Input: part model. Units: mm. Frame: model coordinates. Round coordinates to 2 decimals unless told otherwise and drop trailing zeros. Write each loop counter-clockwise with the first axis right and the second up, starting at its lowest first coordinate (ties: lowest second). Pieces come first, ordered by that corner, then holes. Notation, with made-up numbers: (17, 17) - (68, 17) arc R13 cw to (68, 26) - close; hole circle Ø9 at (61, 4). An arc over 180 degrees is marked (long way). Use one line per item in the form item = value.
```python
from build123d import *

# Parameters (mm, degrees)
SKETCH1_W           = 128
SKETCH1_H           = 90
SKETCH1_R           = 2.4
SKETCH1_R_2         = 1.5
BOSS_EXTRUDE3_DEPTH = 10


with BuildPart() as part:
    # Sketch1 → Boss-Extrude3 (new body)
    with BuildSketch(Plane.XY):
        with Locations((-55.79, 35.875)):
            Rectangle(SKETCH1_W, SKETCH1_H)
        with Locations((0, 71.73)):
            Circle(SKETCH1_R, mode=Mode.SUBTRACT)
        with Locations((-111.58, 0)):
            Circle(SKETCH1_R, mode=Mode.SUBTRACT)
        Circle(SKETCH1_R, mode=Mode.SUBTRACT)
        with Locations((-111.58, 71.73)):
            Circle(SKETCH1_R, mode=Mode.SUBTRACT)
        with Locations((-97.694375804, 60.375)):
            Circle(SKETCH1_R_2, mode=Mode.SUBTRACT)
        with Locations((-39.694375804, 60.375)):
            Circle(SKETCH1_R_2, mode=Mode.SUBTRACT)
        with Locations((-39.694375804, 11.375)):
            Circle(SKETCH1_R_2, mode=Mode.SUBTRACT)
        with Locations((-97.694375804, 11.375)):
            Circle(SKETCH1_R_2, mode=Mode.SUBTRACT)
    extrude(amount=BOSS_EXTRUDE3_DEPTH)


solid = part.part
```
(1) Draft query along X for faces 1 (the face through (-57, 37, 10)), 2 (the face through (1.29, 2.024, 4.93)), 3 (the face through (8.21, 35, 5)). Return one class per face: released by +X, released by -X, zero draft, split by the parting line, or undercut.
Derived:
face_1 = zero draft
face_2 = undercut
face_3 = released by +X
(2) First-contact query: pin 1 Ø5 at (x, y) = (-97.69, 11.38) entering from +Z; pin 2 Ø4.5 at (x, y) = (-111.58, 71.73) entering from -Z. Flat tips, straight axial feed; report the tip coordinate or a pass-through.
Derived:
pin_1 = 10
pin_2 = through
(3) Material intervals for L1, parallel to Y at x = -111.5, z = 5.75 (3 decimals); L2, parallel to X at y = 59.5, z = 3.25; L3, parallel to X at y = -2, z = 8.5, sorted ascending.
Derived:
L1 = -9.125 to -2.399, 2.399 to 69.331, 74.129 to 80.875
L2 = -119.79 to -98.91, -96.48 to -40.91, -38.48 to 8.21
L3 = -119.79 to -112.91, -110.25 to -1.33, 1.33 to 8.21
(4) Cut plane A-A on y = 0. Output: boundary loops of the cut face in (x, z).
Derived:
outline = (-119.79, 0) - (-113.98, 0) - (-113.98, 10) - (-119.79, 10) - close; (-109.18, 0) - (-2.4, 0) - (-2.4, 10) - (-109.18, 10) - close; (2.4, 0) - (8.21, 0) - (8.21, 10) - (2.4, 10) - close
(5) Cut plane B-B on x = -111.58. Output: boundary loops of the cut face in (y, z) (3 decimals), then the cut area to 3 significant figures.
Derived:
outline = (-9.125, 0) - (-2.4, 0) - (-2.4, 10) - (-9.125, 10) - close; (2.4, 0) - (69.33, 0) - (69.33, 10) - (2.4, 10) - close; (74.13, 0) - (80.875, 0) - (80.875, 10) - (74.13, 10) - close
area = 804 mm^2
